For this review, take the finished solid that the model builds, in its own axes (mm). Round coordinates to 2 decimals unless told otherwise and drop trailing zeros. Loops run counter-clockwise (first coordinate to the right, second up) from the corner with the lowest first, then second, coordinate; pieces in that order, holes last. Notation, with made-up numbers: M 29,-33.75 L 56,-33.75 A23 ccw 56,-17.75 Z; hole C 74,-36.5 d8. An arc over 180 degrees is marked long. One line per question, with ' | ' between items. Start each with the question number.
1) For probe 1 along X at (y, z) = (-3, 190.5); probe 2 along Z at (x, y) = (6.25, 3); probe 3 along Z at (x, y) = (-6, -16), list the stretches that pass through material, from the lowest coordinate up. Write a range as from..to.
2) For pin 1 Ø5 at (y, z) = (14, 54) entering from -X; pin 2 Ø10 at (x, y) = (6, 6.5) entering from +Z, all flat-tipped, find the tip position at first contact; note any pin that passes through.
3) We need section D-D (y = 9.5). Give the boundary of the cut face in (x, z), and give its area (3 significant figures).
4) We need section C-C (x = 4.25). Give the boundary of the cut face in (y, z).
5) We need section B-B (z = 77). Give the boundary of the cut face in (x, y).
6) We need section A-A (y = 0). Give the boundary of the cut face in (x, z).
```python
from build123d import *

# Parameters (mm, degrees)
EXTRUDE_1_DEPTH = 20
SKETCH_2_R      = 30
EXTRUDE_2_DEPTH = 10


with BuildPart() as part:
    # 草图1 → 凸台-拉伸1 (new body)
    with BuildSketch(Plane(origin=(0, 0, 0), x_dir=(0, 0, -1), z_dir=(1, 0, 0))):
        with BuildLine():
            Line((0, 30), (-200, 30))
            ThreePointArc((-200, 30), (-230, 0), (-200, -30))
            Line((-200, -30), (0, -30))
            ThreePointArc((0, -30), (30, 0), (0, 30))
        make_face()
    extrude(amount=EXTRUDE_1_DEPTH)

    # 草图2 → 凸台-拉伸2 (add)
    with BuildSketch(Plane.ZY):
        Circle(SKETCH_2_R)
    extrude(amount=EXTRUDE_2_DEPTH)


solid = part.part
```
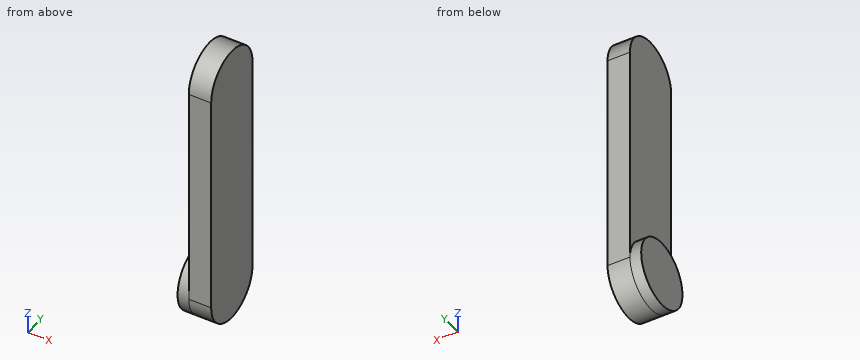
Answers below:
1) probe 1: 0..20 | probe 2: -29.85..229.85 | probe 3: -25.38..25.38
2) pin 1: x = 0 | pin 2: z = 229.96
3) outline: M -10,-28.46 L 20,-28.46 L 20,228.46 L 0,228.46 L 0,28.46 L -10,28.46 Z | area: 5,710 mm^2
4) outline: M -30,0 A30 ccw 30,0 L 30,200 A30 ccw -30,200 Z
5) outline: M 0,-30 L 20,-30 L 20,30 L 0,30 Z
6) outline: M -10,-30 L 20,-30 L 20,230 L 0,230 L 0,30 L -10,30 Z
